from build123d import *

# Parameters (mm, degrees)
F1_DEPTH = 80


with BuildPart() as f1:
    # F0 (on Top) → F1 (new body)
    with BuildSketch(Plane.XY):
        with BuildLine():
            ThreePointArc((-33.671542, 20.483526), (-32.829683, 21.325384), (-31.679683, 21.633526))
            Line((-31.679683, 21.633526), (27.720317, 21.633526))
            ThreePointArc((27.720317, 21.633526), (28.870317, 21.325384), (29.712175, 20.483526))
            Line((29.712175, 20.483526), (61.387175, -34.379184))
            Line((61.387175, -34.379184), (63.119226, -33.379184))
            Line((63.119226, -33.379184), (31.444226, 21.483526))
            ThreePointArc((31.444226, 21.483526), (29.870317, 23.057435), (27.720317, 23.633526))
            Line((27.720317, 23.633526), (-31.679683, 23.633526))
            ThreePointArc((-31.679683, 23.633526), (-33.829683, 23.057435), (-35.403592, 21.483526))
            Line((-35.403592, 21.483526), (-67.078592, -33.379184))
            Line((-67.078592, -33.379184), (-65.346542, -34.379184))
            Line((-65.346542, -34.379184), (-33.671542, 20.483526))
        make_face()
    extrude(amount=F1_DEPTH)


solid = f1.part
Input: part model. Units: mm. Frame: model coordinates. A direction names the side the tool comes from. Round coordinates to 2 decimals unless told otherwise and drop trailing zeros. Order: outer loops, then holes, each group sorted by start corner. A loop starts at its lowest first (then second) coordinate and runs counter-clockwise, first axis right, second up.
1. Cut plane B-B, the plane y = 14. Output: boundary loops of the cut face in (x, z).
The answers:
outline: (-39.72, 0) - (-37.41, 0) - (-37.41, 80) - (-39.72, 80) - close; (33.46, 0) - (35.76, 0) - (35.76, 80) - (33.46, 80) - close
2. Cut plane C-C, the plane x = -19. Output: boundary loops of the cut face in (y, z), then the cut area to 3 significant figures.
The answers:
outline: (21.63, 0) - (23.63, 0) - (23.63, 80) - (21.63, 80) - close
area: 160 mm2
3. Pin query (flat end, axial travel): P1, Ø2, axis at x = -25, z = 39.5, coming from the -Y side; P2, Ø4, axis at x = 32.5, z = 68, coming from the -Y side; P3, Ø8, axis at y = 4.5, z = 13, coming from the +X side. Return the tip coordinate at first contact, or that it passes through.
The answers:
P1: stops at y = 21.63
P2: stops at y = 12.19
P3: stops at x = 43.56
4. Cut plane A-A, the plane z = 5.5. Output: boundary loops of the cut face in (x, y).
The answers:
outline: (-67.08, -33.38) - (-65.35, -34.38) - (-33.67, 20.48) arc R2.3 cw to (-31.68, 21.63) - (27.72, 21.63) arc R2.3 cw to (29.71, 20.48) - (61.39, -34.38) - (63.12, -33.38) - (31.44, 21.48) arc R4.3 ccw to (27.72, 23.63) - (-31.68, 23.63) arc R4.3 ccw to (-35.4, 21.48) - close
5. Set-up query: faces 1 (the face through (47.503, -6.332, 39.44)), 2 (the face through (45.328, -6.564, 39.44)). Return all of +Z, -Z, +X, -X, +Y, -Y with unobstructed straight access to the full face (end or side cutting, diameter ignored); none if empty.
The answers:
face 1: +Z, -Z, +X, +Y
face 2: +Z, -Z, -Y
6. Mould query, pull axis X, two halves, no side actions, for faces 3 (the face through (-33.802, 23.073, 39.44)), 4 (the face through (-2, 23, 0)), 5 (the face through (-49.73, -7.33, 39.44)). Classes: released by +X, released by -X, zero draft, split by the parting line, or undercut.
The answers:
face 3: released by -X
face 4: zero draft
face 5: undercut
7. Material intervals for line 1 (Y direction, x = 20, z = 40.5); line 2 (X direction, y = -3.5, z = 70.5); line 3 (X direction, y = 2, z = 6.5), sorted ascending.
The answers:
line 1: y = 21.63 to 23.63
line 2: x = -49.83 to -47.52, 43.56 to 45.87
line 3: x = -46.65 to -44.34, 40.38 to 42.69
8. Cut plane D-D, the plane x = -50. Output: boundary loops of the cut face in (y, z).
The answers:
outline: (-7.8, 0) - (-3.8, 0) - (-3.8, 80) - (-7.8, 80) - close
